```python
from build123d import *

# Parameters (mm, degrees)
SKETCH1_R               = 7.5565
BOSS_EXTRUDE1_DEPTH     = 29.2608
SKETCH2_R               = 11.2776
BOSS_EXTRUDE2_DEPTH     = 11.78052
SKETCH3_R               = 9.02208
BOSS_EXTRUDE3_DEPTH     = 7.63524
CUT_EXTRUDE1_DEPTH      = 52.222807586
CUT_EXTRUDE1_DEPTH_BACK = 52.222807586
SKETCH4_R               = 1.5875


with BuildPart() as part:
    # Sketch1 → Boss-Extrude1 (new body)
    with BuildSketch(Plane(origin=(0, 0, 0), x_dir=(1, 0, 0), z_dir=(0, 1, 0))):
        with Locations(Location((0, 0, 0), (0, 0, 270))):
            Circle(SKETCH1_R)
    extrude(amount=BOSS_EXTRUDE1_DEPTH)

    # Sketch2 → Boss-Extrude2 (add)
    with BuildSketch(Plane(origin=(0, 29.2608, 0), x_dir=(1, 0, 0), z_dir=(0, 1, 0))):
        with Locations(Location((0, 0, 0), (0, 0, 90))):
            Circle(SKETCH2_R)
    extrude(amount=BOSS_EXTRUDE2_DEPTH)

    # Sketch3 → Boss-Extrude3 (add)
    with BuildSketch(Plane(origin=(0, 41.04132, 0), x_dir=(1, 0, 0), z_dir=(0, 1, 0))):
        with Locations(Location((0, 0, 0), (0, 0, 90))):
            Circle(SKETCH3_R)
    extrude(amount=BOSS_EXTRUDE3_DEPTH)

    # Sketch4 → Cut-Extrude1 (cut, two sides: drawn at the far end of the back side and taken through both)
    with BuildSketch(Plane.XY.offset(-CUT_EXTRUDE1_DEPTH_BACK)):
        with Locations((0.06604, 3.402959253)):
            Circle(SKETCH4_R)
    extrude(amount=CUT_EXTRUDE1_DEPTH + CUT_EXTRUDE1_DEPTH_BACK, mode=Mode.SUBTRACT)


solid = part.part
```
Input: part model. Units: mm. Frame: model coordinates. A direction names the side the tool comes from. Coordinates: 2 decimals unless noted, no trailing zeros. Order: outer loops, then holes, each group sorted by start corner. A loop starts at its lowest first (then second) coordinate and runs counter-clockwise, first axis right, second up. Notation, with made-up numbers: (-6, 89.5) - (41, 89.5) arc R25 ccw to (41, 113.5) - close; hole circle Ø9 at (88, 80). An arc over 180 degrees is marked (long way). Return JSON: item names as keys, results as strings.
Q1. Cut plane B-B (x = 0). Return loops of the section in (y, z).
The answers:
{"outline": "(0, -7.56) - (1.82, -7.56) - (1.82, 7.56) - (0, 7.56) - close; (4.99, -7.56) - (29.26, -7.56) - (29.26, -11.28) - (41.04, -11.28) - (41.04, -9.02) - (48.68, -9.02) - (48.68, 9.02) - (41.04, 9.02) - (41.04, 11.28) - (29.26, 11.28) - (29.26, 7.56) - (4.99, 7.56) - close"}
Q2. Cut plane C-C (y = 12.5). Return loops of the section in (x, z), then the cut area to 3 significant figures.
The answers:
{"outline": "circle Ø15.11 at (0, 0)", "area": "179 mm2"}
Q3. Access query for faces 4 (the flat face through (0, 0, 0)), 5 (the flat face through (-8, 41.041, 5)). Directions: +Z, -Z, +X, -X, +Y, -Y. A direction counts if a zero-diameter tool reaches every point of the face in a straight line with its end or side. Return the directions, or none.
The answers:
{"face 4": "+Z, -Z, +X, -X, -Y", "face 5": "+Y"}
Q4. First-contact query: pin 1 (4 mm diameter, centred on y = 37.5, z = -4, fed in from +X); pin 2 (5 mm diameter, centred on y = 41, z = -3.5, fed in from -X); pin 3 (12 mm diameter, centred on x = -1.5, z = 8.5, fed in from -Y); pin 4 (3 mm diameter, centred on y = 10.5, z = 3, fed in from +X). Flat tips, straight axial feed; report the tip coordinate or a pass-through.
The answers:
{"pin 1": "stops at x = 11.1", "pin 2": "stops at x = -11.23", "pin 3": "stops at y = 0", "pin 4": "stops at x = 7.41"}
Q5. Ray query, probe 1 along Y at (x, z) = (-4.25, 7.25); probe 2 along Y at (x, z) = (5, -8); probe 3 along X at (y, z) = (3, 6.5). Return the intervals inside material, ascending.
The answers:
{"probe 1": "y = 29.26 to 48.68", "probe 2": "y = 29.26 to 41.04", "probe 3": "x = -3.85 to -1.47, 1.6 to 3.85"}
Q6. Cut plane D-D (z = -2). Return loops of the section in (x, y) (1 decimal).
The answers:
{"outline": "(-11.1, 29.3) - (-7.3, 29.3) - (-7.3, 0) - (7.3, 0) - (7.3, 29.3) - (11.1, 29.3) - (11.1, 41) - (8.8, 41) - (8.8, 48.7) - (-8.8, 48.7) - (-8.8, 41) - (-11.1, 41) - close; hole circle Ø3.2 at (0.1, 3.4)"}
Q7. Cut plane A-A (z = 2.75). Return loops of the section in (x, y) (1 decimal).
The answers:
{"outline": "(-10.9, 29.3) - (-7, 29.3) - (-7, 0) - (7, 0) - (7, 29.3) - (10.9, 29.3) - (10.9, 41) - (8.6, 41) - (8.6, 48.7) - (-8.6, 48.7) - (-8.6, 41) - (-10.9, 41) - close; hole circle Ø3.2 at (0.1, 3.4)"}
Q8. Draft query along X for faces 1 (the cylindrical face through (2.3, 14.4, 7.2)), 2 (the cylindrical face through (-0.278, 1.853, -0.107)), 3 (the flat face through (2.3, 29.261, -7.4)). Return one class per face: +X half, -X half, draft (parallel to the pull), parting line (faces both ways), or undercut.
The answers:
{"face 1": "parting line", "face 2": "undercut", "face 3": "draft"}
